Design review of the part built by this model. Coordinates are the model's own, in mm. A direction names the side the tool comes from. Round coordinates to 2 decimals unless told otherwise and drop trailing zeros. Order: outer loops, then holes, each group sorted by start corner. A loop starts at its lowest first (then second) coordinate and runs counter-clockwise, first axis right, second up. Notation, with made-up numbers: M -31,-14 L 10,-14 A16 cw 10,3 Z; hole C 12,28.5 d2. An arc over 180 degrees is marked long. Write each question's results on one line, items separated by ' | '. Start each with the question number.
Item 1: Machinability: for faces 4 (the flat face through (2.93, 7.14, -0.28)), 5 (the flat face through (-20.595, 13.969, -2.965)), 6 (the flat face through (-23, 15, 2.75)), which of the approach directions +Z, -Z, +X, -X, +Y, -Y give a long, thin tool a straight path to every point of the face, cutting with its end or side? Answer none if there is none.
Item 2: Take a section at B-B, the plane y = 14.25. Write out the cut boundary in (x, z), plus the area to 3 significant figures.
Item 3: Take a section at C-C, the plane y = 6. Write out the cut boundary in (x, z).
Item 4: Clearance check with flat-ended pins moving along their axes: pin 1 (1.8 mm diameter, centred on x = -22.43, y = 16.1, fed in from -Z); pin 2 (3 mm diameter, centred on x = -5.5, y = 10.5, fed in from -Z); pin 3 (1 mm diameter, centred on y = 10, z = 1, fed in from +X); pin 4 (4.5 mm diameter, centred on x = -5, y = 9.5, fed in from +Z). State where each tip first meets the part, or that it passes through.
Item 5: Take a section at D-D, the plane x = -3.75. Write out the cut boundary in (y, z), plus the area to 3 significant figures.
Item 6: Wall thickness on line 1 (Y direction, x = -0.5, z = -0.45); line 2 (Y direction, x = -23, z = 2.55); line 3 (Y direction, x = -1.75, z = -1.1): over which ranges is each line inside the solid? List them lowest first. Write a range as [from, to].
Item 7: The part is to be moulded in two halves that separate along Y. For faces 1 (the cylindrical face through (-23.17, 16.77, -3)), 2 (the cylindrical face through (-22.728, 12.761, 2.107)), 3 (the flat face through (-23, 15, 2.25)), say which applies: +Y half, -Y half, draft (parallel to the pull), parting line (faces both ways), or undercut.
Item 8: Take a section at A-A, the plane z = -1.4. Write out the cut boundary in (x, y), plus the area to 3 significant figures.
```python
from build123d import *

# Parameters (mm, degrees)
ODGI_CIE_BAZOWE1_DEPTH      = 1.75
ODGI_CIE_BAZOWE1_DEPTH_BACK = 2.25
WYTNIJ_WYCI_GNI_CIE1_REACH  = 28.618
ODGI_CIE_KRAW_DZI1_DEPTH    = 4
ODGI_CIE_KRAW_DZI2_DEPTH    = 4
SZKIC13_R                   = 1
WYTNIJ_WYCI_GNI_CIE2_DEPTH  = 32.329703674
ZAOKR_GLENIE1_R             = 2


# Sheet-metal steps are written as plain solids
with BuildPart() as part:
    # Szkic1 → Odgięcie bazowe1 (new, two sides: drawn at the far end of the back side and taken through both)
    with BuildSketch(Plane.XY.offset(-ODGI_CIE_BAZOWE1_DEPTH_BACK)):
        with BuildLine():
            Line((-24.746406247, 12.272623445), (2.164511805, 10.081165123))
            ThreePointArc((2.164511805, 10.081165123), (2.845512893, 9.731845847), (3.080047351, 9.003299331))
            Line((3.080047351, 9.003299331), (2.773055226, 5.233462675))
            ThreePointArc((2.773055226, 5.233462675), (2.42373595, 4.552461587), (1.695189434, 4.317927129))
            Line((1.695189434, 4.317927129), (-0.581165123, 4.503299331))
            ThreePointArc((-0.581165123, 4.503299331), (-1.177803392, 6.235243199), (0.5, 5.5))
            Line((0.5, 5.5), (1, 5.5))
            ThreePointArc((1, 5.5), (-1.516705088, 6.602864798), (-0.621747685, 4.004948997))
            Line((-0.621747685, 4.004948997), (1.654606873, 3.819576795))
            ThreePointArc((1.654606873, 3.819576795), (2.747426646, 4.171378482), (3.27140556, 5.192880113))
            Line((3.27140556, 5.192880113), (3.578397685, 8.96271677))
            ThreePointArc((3.578397685, 8.96271677), (3.226595998, 10.055536543), (2.205094367, 10.579515457))
            Line((2.205094367, 10.579515457), (-24.705823686, 12.77097378))
            Line((-24.705823686, 12.77097378), (-24.746406247, 12.272623445))
        make_face()
    extrude(amount=ODGI_CIE_BAZOWE1_DEPTH + ODGI_CIE_BAZOWE1_DEPTH_BACK)

    # Szkic6 → Wytnij-wyciągnięcie1 (cut, up to next)
    with BuildSketch(Plane(origin=(0.870381249, 10.688206219, 0), x_dir=(0.9967006686068912, -0.08116512304294364, 0), z_dir=(0.08116512304294363, 0.9967006686068911, 0)), mode=Mode.PRIVATE) as wytnij_wyci_gni_cie1_sk1:
        with BuildLine():
            Line((-20.460868644, -1.75), (-21.660868644, -1.75))
            ThreePointArc((-21.660868644, -1.75), (-21.060868644, -1.55), (-20.460868644, -1.75))
        make_face()
    wytnij_wyci_gni_cie1_tool1 = extrude(wytnij_wyci_gni_cie1_sk1.sketch, amount=-WYTNIJ_WYCI_GNI_CIE1_REACH, mode=Mode.PRIVATE) & part.part
    # Szkic6 → Wytnij-wyciągnięcie1 (cut, up to next)
    with BuildSketch(Plane(origin=(0.870381249, 10.688206219, 0), x_dir=(0.9967006686068912, -0.08116512304294364, 0), z_dir=(0.08116512304294363, 0.9967006686068911, 0)), mode=Mode.PRIVATE) as wytnij_wyci_gni_cie1_sk2:
        with BuildLine():
            Line((-20.460868644, 2.25), (-21.660868644, 2.25))
            ThreePointArc((-21.660868644, 2.25), (-21.060868644, 2.05), (-20.460868644, 2.25))
        make_face()
    wytnij_wyci_gni_cie1_tool2 = extrude(wytnij_wyci_gni_cie1_sk2.sketch, amount=-WYTNIJ_WYCI_GNI_CIE1_REACH, mode=Mode.PRIVATE) & part.part
    add(wytnij_wyci_gni_cie1_tool1.solids().sort_by_distance((-20.121001, 12.397614, 1.669272))[0], mode=Mode.SUBTRACT)
    add(wytnij_wyci_gni_cie1_tool2.solids().sort_by_distance((-20.121001, 12.397614, -2.169272))[0], mode=Mode.SUBTRACT)

    # Odgięcie krawędzi1 section (across the edge) → Odgięcie krawędzi1 (add)
    with BuildSketch(Plane(origin=(-24.705823686, 12.77097378, 2.25), x_dir=(0, 0, -1), z_dir=(0.9967006686068913, -0.08116512304294192, 0))):
        with BuildLine():
            Line((-0.5, 0.5), (-0.5, 5.5))
            Line((-0.5, 5.5), (0, 5.5))
            Line((0, 5.5), (0, 0.5))
            ThreePointArc((0, 0.5), (0.146446609, 0.146446609), (0.5, 0))
            Line((0.5, 0), (0.5, -0.5))
            ThreePointArc((0.5, -0.5), (-0.207106781, -0.207106781), (-0.5, 0.5))
        make_face()
    extrude(amount=ODGI_CIE_KRAW_DZI1_DEPTH)

    # Odgięcie krawędzi2 section (across the edge) → Odgięcie krawędzi2 (add)
    with BuildSketch(Plane(origin=(-20.719021011, 12.446313287, -2.75), x_dir=(0, 0, 1), z_dir=(-0.9967006686068913, 0.08116512304294192, 0))):
        with BuildLine():
            Line((-0.5, 0.5), (-0.5, 5.5))
            Line((-0.5, 5.5), (0, 5.5))
            Line((0, 5.5), (0, 0.5))
            ThreePointArc((0, 0.5), (0.146446609, 0.146446609), (0.5, 0))
            Line((0.5, 0), (0.5, -0.5))
            ThreePointArc((0.5, -0.5), (-0.207106781, -0.207106781), (-0.5, 0.5))
        make_face()
    extrude(amount=ODGI_CIE_KRAW_DZI2_DEPTH)

    # Szkic13 → Wytnij-wyciągnięcie2 (cut, through all)
    with BuildSketch(Plane.XY.offset(2.75)):
        with Locations((-22.428344418, 16.097095874)):
            Circle(SZKIC13_R)
    extrude(amount=-WYTNIJ_WYCI_GNI_CIE2_DEPTH, mode=Mode.SUBTRACT)

    # Zaokrąglenie1
    zaokr_glenie1_edges = [part.edges().sort_by_distance(p)[0] for p in [
        (-24.259415509, 18.252827457, -3),
        (-20.272612835, 17.928166965, -3),
        (-20.272612835, 17.928166965, 2.5),
        (-24.259415509, 18.252827457, 2.5),
    ]]
    fillet(zaokr_glenie1_edges, radius=ZAOKR_GLENIE1_R - 0.0001)  # a hair under: the kernel refuses the full size


solid = part.part
```
Results list:
1) face 4: +Z, -Z | face 5: -Z, +X, -Y | face 6: +Z, +X, -X, +Y, -Y
2) outline: M -24.59,-3.25 L -20.57,-3.25 L -20.57,-2.75 L -24.59,-2.75 Z; M -24.59,2.25 L -20.57,2.25 L -20.57,2.75 L -24.59,2.75 Z | area: 4.01 mm²
3) outline: M -1.91,-2.25 L -1.37,-2.25 L -1.37,1.75 L -1.91,1.75 Z; M 0.37,-2.25 L 0.91,-2.25 L 0.91,1.75 L 0.37,1.75 Z; M 2.84,-2.25 L 3.34,-2.25 L 3.34,1.75 L 2.84,1.75 Z
4) pin 1: through | pin 2: z = -2.25 | pin 3: x = 3.52 | pin 4: z = 1.75
5) outline: M 10.56,-2.25 L 11.06,-2.25 L 11.06,1.75 L 10.56,1.75 Z | area: 2.01 mm²
6) line 1: [4, 4.5], [6.5, 7], [10.3, 10.8] | line 2: [12.53, 15.28], [16.92, 18.01] | line 3: [4.67, 6.33], [10.4, 10.9]
7) face 1: undercut | face 2: +Y half | face 3: draft
8) outline: M -24.75,12.27 L 2.16,10.08 A1 cw 3.08,9 L 2.77,5.23 A1 cw 1.7,4.32 L -0.58,4.5 A1 cw long 0.5,5.5 L 1,5.5 A1.5 ccw long -0.62,4 L 1.65,3.82 A1.5 ccw 3.27,5.19 L 3.58,8.96 A1.5 ccw 2.21,10.58 L -24.71,12.77 Z | area: 21.4 mm²
